Model file for the job. Use its own axes, mm. A direction names the side the tool comes from. Round coordinates to 2 decimals unless told otherwise and drop trailing zeros. Order: outer loops, then holes, each group sorted by start corner. A loop starts at its lowest first (then second) coordinate and runs counter-clockwise, first axis right, second up. Notation, with made-up numbers: (24.25, -29) - (67.25, -29) arc R25 ccw to (67.25, -4) - close; hole circle Ø6 at (6, 73.25). An arc over 180 degrees is marked (long way). Put each result on its own line as item: value. Start each with the question number.
Item 1: Which spindle directions (+Z, -Z, +X, -X, +Y, -Y) get a long thin tool onto all of the face, cutting with end or side? Do faces 1 (the face through (4.9, 0.1, 1.2)), 2 (the face through (7.469, 9.5, 0.6)), 3 (the face through (5, 4, 1)). Say none if no direction does.
Item 2: Saw through at D-D on z = 2.7. List the corners of the cut face in (x, y).
Item 3: Saw through at A-A on x = 4. List the corners of the cut face in (y, z).
Item 4: Probe probe 1 along Z at (x, y) = (2, 7); probe 2 along X at (y, z) = (2.25, 4.15); probe 3 along Y at (x, z) = (0.5, 3.3). List the from-to ranges inside material, lowest first.
Item 5: Saw through at C-C on y = 6.5. List the corners of the cut face in (x, z).
Item 6: Saw through at B-B on z = 0.65. List the corners of the cut face in (x, y).
Item 7: Mould opens along Y. For faces 4 (the face through (4.93, 9.91, 2.92)), 5 (the face through (8.216, 6.535, 0.641)), 6 (the face through (5, 0, 3)) say: pulls with the +Y half, pulls with the -Y half, needs draft (parallel to the pull), parting line crosses it, or undercut.
Item 8: Pin check, flat tips, straight feed: pin 1 Ø0.5 at (y, z) = (9.5, 1) entering from +X; pin 2 Ø1.8 at (x, y) = (5.5, 6) entering from -Z; pin 3 Ø1.4 at (x, z) = (5, 0.5) entering from +Y. Stop position of each tip, or through.
```python
from build123d import *

# Parameters (mm, degrees)
SKETCH1_W           = 10
SKETCH1_H           = 10
BOSS_EXTRUDE1_DEPTH = 4.5
CHAMFER1_SIZE       = 2.9
CHAMFER1_SIZE2      = 0.2
CHAMFER3_SIZE       = 0.18787374
CHAMFER3_SIZE_2     = 5.38
CHAMFER4_SIZE       = 0.3
CUT_EXTRUDE1_DEPTH  = 1.3
CHAMFER5_SIZE       = 0.2
CHAMFER5_SIZE2      = 2.4


with BuildPart() as part:
    # Sketch1 → Boss-Extrude1 (new body)
    with BuildSketch(Plane.XY):
        with Locations((5, 5)):
            Rectangle(SKETCH1_W, SKETCH1_H)
    extrude(amount=BOSS_EXTRUDE1_DEPTH)

    # Chamfer1
    chamfer1_edges = [part.edges().sort_by_distance(p)[0] for p in [
        (5, 10, 4.5),
    ]]
    chamfer1_side = [part.faces().sort_by_distance(p)[0] for p in [
        (5, 10, 2.25),
    ]]
    chamfer(chamfer1_edges, length=CHAMFER1_SIZE, length2=CHAMFER1_SIZE2, reference=chamfer1_side[0])

    # Chamfer3
    # the kernel refuses this chamfer: 5.38, 0.18787374 mm, written as the material it takes off along each edge
    with BuildSketch(Plane(origin=(0, 23.787684867, 4.5), x_dir=(0.6724220033128364, 0, 0.7401679873250072), z_dir=(0, -1, 0))) as chamfer3_piece_1:
        Polygon((CHAMFER3_SIZE * 0.672422002832, -CHAMFER3_SIZE * 0.740167986796), (-CHAMFER3_SIZE_2 * 0.740167987325, -CHAMFER3_SIZE_2 * 0.672422003313), (0, 0), align=None)
    extrude(amount=37.775369733, mode=Mode.SUBTRACT)
    with BuildSketch(Plane(origin=(10, -13.987684867, 4.5), x_dir=(0.0013423185755924109, 0, -0.999999099090015), z_dir=(0, 1, 0))) as chamfer3_piece_2:
        Polygon((CHAMFER3_SIZE_2 * 0.99999909909, CHAMFER3_SIZE_2 * 0.00134231857559), (-CHAMFER3_SIZE * 0.00134231857463, CHAMFER3_SIZE * 0.999999098375), (0, 0), align=None)
    extrude(amount=37.775369733, mode=Mode.SUBTRACT)

    # Chamfer4
    chamfer4_edges = [part.edges().sort_by_distance(p)[0] for p in [
        (5, 9.8, 4.5),
        (5, 0, 4.5),
        (9.81212626, 4.9, 4.5),
        (0.18787374, 4.9, 4.5),
    ]]
    chamfer(chamfer4_edges, length=CHAMFER4_SIZE)

    # Sketch2 → Cut-Extrude1 (cut)
    with BuildSketch(Plane(origin=(0, 0, 0), x_dir=(-1, 0, 0), z_dir=(0, 0, -1))):
        Polygon((-7.469269723, 10), (-7.469269723, 9), (-7.969269723, 9), (-8.469269723, 4), (-1.530730277, 4), (-2.030730277, 9), (-2.530730277, 9), (-2.530730277, 10), align=None)
    extrude(amount=-CUT_EXTRUDE1_DEPTH, mode=Mode.SUBTRACT)

    # Chamfer5
    chamfer5_edges = [part.edges().sort_by_distance(p)[0] for p in [
        (5, 0, 0),
    ]]
    chamfer5_side = [part.faces().sort_by_distance(p)[0] for p in [
        (5, 3.900810123, 0),
    ]]
    chamfer(chamfer5_edges, length=CHAMFER5_SIZE, length2=CHAMFER5_SIZE2, reference=chamfer5_side[0])


solid = part.part
```
Results found:
1. face 1: -Z, +X, -X, -Y
1. face 2: -Z, +Y
1. face 3: -Z
2. outline: (0.13, 0) - (9.87, 0) - (9.87, 9.92) - (0.13, 9.92) - close
3. outline: (0, 2.4) - (0.2, 0) - (4, 0) - (4, 1.3) - (10, 1.3) - (10, 1.6) - (9.82, 4.2) - (9.5, 4.5) - (0.3, 4.5) - (0, 4.2) - close
4. probe 1: z = 1.3 to 4.5
4. probe 2: x = 0.18 to 9.82
4. probe 3: y = 0 to 9.88
5. outline: (0.03, 0) - (1.78, 0) - (1.78, 1.3) - (8.22, 1.3) - (8.22, 0) - (9.97, 0) - (9.82, 4.2) - (9.51, 4.5) - (0.49, 4.5) - (0.18, 4.2) - close
6. outline: (0.05, 0.15) - (9.95, 0.15) - (9.95, 10) - (7.47, 10) - (7.47, 9) - (7.97, 9) - (8.47, 4) - (1.53, 4) - (2.03, 9) - (2.53, 9) - (2.53, 10) - (0.05, 10) - close
7. face 4: pulls with the +Y half
7. face 5: undercut
7. face 6: pulls with the -Y half
8. pin 1: stops at x = 9.94
8. pin 2: stops at z = 1.3
8. pin 3: stops at y = 4
